```python
from build123d import *

# Parameters (mm, degrees)
F0_W      = 75
F0_H      = 75
F1_DEPTH  = 60
F2_W      = 55
F2_H      = 30
F3_DEPTH  = 75.001
F5_DEPTH  = 25
F6_R      = 2.1
F7_DEPTH  = 40
F8_R      = 4.1
F9_DEPTH  = 20
F11_DEPTH = 25
F13_DEPTH = 5
F14_R     = 2.1
F15_DEPTH = 15


with BuildPart() as f1:
    # F0 (on Top) → F1 (new body)
    with BuildSketch(Plane.XY):
        Rectangle(F0_W, F0_H)
    extrude(amount=F1_DEPTH)

    # F2 (on face) → F3 (cut, through all)
    with BuildSketch(Plane(origin=(-37.5, 0, 0), x_dir=(0, -1, 0), z_dir=(-1, 0, 0))):
        with Locations((10, 35)):
            Rectangle(F2_W, F2_H)
    extrude(amount=-F3_DEPTH, mode=Mode.SUBTRACT)

    # F4 (on face) → F5 (cut)
    with BuildSketch(Plane(origin=(0, 0, 0), x_dir=(1, 0, 0), z_dir=(0, 0, -1))):
        with BuildLine():
            Line((-12.5, 37.5), (-12.5, 25.976177))
            ThreePointArc((-12.5, 25.976177), (-11.5, -16), (-10.5, 25.976177))
            Line((-10.5, 25.976177), (-10.5, 37.5))
            Line((-10.5, 37.5), (-12.5, 37.5))
        make_face()
    extrude(amount=-F5_DEPTH, mode=Mode.SUBTRACT)

    # F6 (on face) → F7 (cut)
    with BuildSketch(Plane(origin=(-37.5, 0, 0), x_dir=(0, -1, 0), z_dir=(-1, 0, 0))):
        with Locations((32.5, 15)):
            Circle(F6_R)
        with Locations((32.5, 5)):
            Circle(F6_R)
    extrude(amount=-F7_DEPTH, mode=Mode.SUBTRACT)

    # F8 (on face) → F9 (cut)
    with BuildSketch(Plane(origin=(-37.5, 0, 0), x_dir=(0, -1, 0), z_dir=(-1, 0, 0))):
        with Locations((32.5, 15)):
            Circle(F8_R)
        with Locations((32.5, 5)):
            Circle(F8_R)
    extrude(amount=-F9_DEPTH, mode=Mode.SUBTRACT)

    # F10 (on face) → F11 (cut)
    with BuildSketch(Plane.XY.offset(60)):
        with BuildLine():
            ThreePointArc((15, 13), (13, 11), (15, 9))
            Line((15, 9), (25, 9))
            ThreePointArc((25, 9), (27, 11), (25, 13))
            Line((25, 13), (15, 13))
        make_face()
        with BuildLine():
            ThreePointArc((15, -19), (13, -21), (15, -23))
            Line((15, -23), (25, -23))
            ThreePointArc((25, -23), (27, -21), (25, -19))
            Line((25, -19), (15, -19))
        make_face()
        with BuildLine():
            Line((15.383265, -17.5), (23.597296, -17.5))
            ThreePointArc((23.597296, -17.5), (36.097296, -5), (23.597296, 7.5))
            Line((23.597296, 7.5), (15.383265, 7.5))
            ThreePointArc((15.383265, 7.5), (2.883265, -5), (15.383265, -17.5))
        make_face()
    extrude(amount=-F11_DEPTH, mode=Mode.SUBTRACT)

    # F12 (on face) → F13 (cut)
    with BuildSketch(Plane.XY.offset(60)):
        with BuildLine():
            Line((15, 23.497423), (15.76653, 23.497423))
            ThreePointArc((15.76653, 23.497423), (15.383265, 23.5), (15, 23.497423))
        make_face()
        with BuildLine():
            Line((72, 23.497423), (15.76653, 23.497423))
            Line((15.76653, 23.497423), (15, 23.497423))
            ThreePointArc((15, 23.497423), (-13.116735, -5), (15, -33.497423))
            Line((15, -33.497423), (15, -33.502577))
            Line((15, -33.502577), (72, -33.502577))
            Line((72, -33.502577), (72, 23.497423))
        make_face()
    extrude(amount=-F13_DEPTH, mode=Mode.SUBTRACT)

    # F14 (on face) → F15 (cut)
    with BuildSketch(Plane(origin=(0, 37.5, 0), x_dir=(-1, 0, 0), z_dir=(0, 1, 0))):
        with Locations((-30, 50)):
            Circle(F14_R)
        with Locations((30, 50)):
            Circle(F14_R)
        with Locations((30, 10)):
            Circle(F14_R)
        with Locations((-30, 10)):
            Circle(F14_R)
    extrude(amount=-F15_DEPTH, mode=Mode.SUBTRACT)


solid = f1.part
```
Check sheet for the modelled part. Datum: model origin and axes. Units: mm. A direction names the side the tool comes from. Coordinates: 2 decimals unless noted, no trailing zeros. Loops run counter-clockwise (first coordinate to the right, second up) from the corner with the lowest first, then second, coordinate; pieces in that order, holes last.
1) Sectioned sample at C-C (x = -20.5). Record the boundary of the cut face in (y, z), and give its area (3 significant figures).
2) Gauge pin test, flat ends, axial feed: pin 1 (5 mm diameter, centred on x = -4, y = -9, fed in from +Z); pin 2 (4 mm diameter, centred on x = 3, z = 40.5, fed in from -Y); pin 3 (5 mm diameter, centred on y = -32.5, z = 15, fed in from -X). Record the tip position at first contact, or that the pin passes through.
3) Sectioned sample at A-A (y = -5). Record the boundary of the cut face in (x, z), and give its area (3 significant figures).
4) Material ranges on probe 1 along Z at (x, y) = (30, 31.75); probe 2 along Z at (x, y) = (-2, -32.5); probe 3 along Z at (x, y) = (-34, 16.5), recorded low to high.
5) Release check for a two-part mould opening along X. For faces 1 (the face through (2.5, -32, 15)), 2 (the face through (20, -23, 53)), 3 (the face through (12, 8, 55)) record: released by +X, released by -X, zero draft, split by the parting line, or undercut.
6) Sectioned sample at D-D (x = -3.5). Record the boundary of the cut face in (y, z), and give its area (3 significant figures).
7) Sectioned sample at B-B (z = 5). Record the boundary of the cut face in (x, y), and give its area (3 significant figures).
8) Access from +Z, -Z, +X, -X, +Y, -Y to the whole of each face (thin tool, end or side, straight path). Record for faces 4 (the face through (-15.04, -30.4, 5.09)), 5 (the face through (30, 22.5, 50)), 6 (the face through (27, 23.497, 58)), 7 (the face through (20, 7.5, 53)).
Check sheet entries:
1. outline: (-37.5, 0) - (-23.97, 0) - (-23.97, 20) - (-37.5, 20) - close; (-37.5, 50) - (17.5, 50) - (17.5, 20) - (13.97, 20) - (13.97, 0) - (37.5, 0) - (37.5, 60) - (-37.5, 60) - close; hole circle Ø8.2 at (-32.5, 5); hole circle Ø8.2 at (-32.5, 15)
1. area: 1,990 mm2
2. pin 1: stops at z = 55
2. pin 2: stops at y = 17.5
2. pin 3: stops at x = -17.5
3. outline: (-37.5, 0) - (-32.5, 0) - (-32.5, 20) - (-37.5, 20) - close; (-37.5, 50) - (2.88, 50) - (2.88, 55) - (-13.12, 55) - (-13.12, 60) - (-37.5, 60) - close; (9.5, 0) - (37.5, 0) - (37.5, 20) - (9.5, 20) - close; (36.1, 50) - (37.5, 50) - (37.5, 55) - (36.1, 55) - close
3. area: 991 mm2
4. probe 1: z = 0 to 7.9, 12.1 to 47.9, 52.1 to 60
4. probe 2: z = 0 to 2.9, 7.1 to 12.9, 17.1 to 20, 50 to 60
4. probe 3: z = 0 to 20, 50 to 60
5. face 1: released by -X
5. face 2: undercut
5. face 3: zero draft
6. outline: (-37.5, 0) - (-24.42, 0) - (-24.42, 20) - (-37.5, 20) - close; (-37.5, 50) - (17.5, 50) - (17.5, 20) - (14.42, 20) - (14.42, 0) - (37.5, 0) - (37.5, 60) - (16.35, 60) - (16.35, 55) - (-26.35, 55) - (-26.35, 60) - (-37.5, 60) - close; hole circle Ø4.2 at (-32.5, 5); hole circle Ø4.2 at (-32.5, 15)
6. area: 1,830 mm2
7. outline: (-37.5, -37.5) - (-12.5, -37.5) - (-12.5, -34.6) - (-17.5, -34.6) - (-17.5, -36.6) - (-37.5, -36.6) - close; (-37.5, -28.4) - (-17.5, -28.4) - (-17.5, -30.4) - (-12.5, -30.4) - (-12.5, -25.98) arc R21 cw (long way) to (-10.5, -25.98) - (-10.5, -30.4) - (2.5, -30.4) - (2.5, -34.6) - (-10.5, -34.6) - (-10.5, -37.5) - (37.5, -37.5) - (37.5, 37.5) - (-37.5, 37.5) - close
7. area: 3,980 mm2
8. face 4: -X
8. face 5: +Y
8. face 6: +Z, +X
8. face 7: +Z
